Part model, mm, in its own coordinate system. Face numbers are marked on the shaded views. A direction names the side the tool comes from. Coordinates: 2 decimals unless noted, no trailing zeros. Write each loop counter-clockwise with the first axis right and the second up, starting at its lowest first coordinate (ties: lowest second). Pieces come first, ordered by that corner, then holes. Notation, with made-up numbers: (50.25, 56) - (89.25, 56) arc R19 ccw to (89.25, 78) - close; hole circle Ø11 at (53, 51.5). An arc over 180 degrees is marked (long way). Use a Markdown table: item, result.
```python
from build123d import *

# Parameters (mm, degrees)
F0_R     = 3.375
F0_R_2   = 20
F1_DEPTH = 15
F2_R     = 31.5
F3_DEPTH = 2
F4_SIZE  = 0.5
F5_SIZE  = 0.5
F6_R     = 23.75
F7_DEPTH = 2.25
F8_SIZE  = 1.5


with BuildPart() as f1:
    # F0 (on Top) → F1 (new body)
    with BuildSketch(Plane.XY):
        with BuildLine():
            ThreePointArc((-102.5, -0.229013), (-90.703842, -28.365124), (-62.500656, -40))
            Line((-62.500656, -40), (62.500656, -40))
            ThreePointArc((62.500656, -40), (90.703842, -28.365124), (102.5, -0.229013))
            Line((102.5, -0.229013), (102.5, 0.229013))
            ThreePointArc((102.5, 0.229013), (90.703842, 28.365124), (62.500656, 40))
            Line((62.500656, 40), (-62.500656, 40))
            ThreePointArc((-62.500656, 40), (-90.703842, 28.365124), (-102.5, 0.229013))
            Line((-102.5, 0.229013), (-102.5, -0.229013))
        make_face()
        with Locations((0, -25.125)):
            Circle(F0_R, mode=Mode.SUBTRACT)
        with Locations((-62.500656, 0)):
            Circle(F0_R_2, mode=Mode.SUBTRACT)
        with Locations((62.500656, 0)):
            Circle(F0_R_2, mode=Mode.SUBTRACT)
        with Locations((0, 25.125)):
            Circle(F0_R, mode=Mode.SUBTRACT)
        with BuildLine():
            ThreePointArc((-102.5, 0.229013), (-102.500656, 0), (-102.5, -0.229013))
            Line((-102.5, -0.229013), (-102.5, 0.229013))
        make_face()
        with BuildLine():
            Line((102.5, 0.229013), (102.5, -0.229013))
            ThreePointArc((102.5, -0.229013), (102.500656, 0), (102.5, 0.229013))
        make_face()
    extrude(amount=F1_DEPTH)

    # F2 (on face) → F3 (cut)
    with BuildSketch(Plane(origin=(0, 0, 0), x_dir=(1, 0, 0), z_dir=(0, 0, -1))):
        with Locations((-62.500656, 0)):
            Circle(F2_R)
        with Locations((62.500656, 0)):
            Circle(F2_R)
    extrude(amount=-F3_DEPTH, mode=Mode.SUBTRACT)

    # F4
    f4_edges = [f1.edges().sort_by_distance(p)[0] for p in [
        (62.500656, 40, 7.5),
        (-62.500656, 40, 7.5),
        (0, 40, 0),
        (0, 40, 15),
    ]]
    chamfer(f4_edges, length=F4_SIZE)

    # F5
    f5_edges = [f1.edges().sort_by_distance(p)[0] for p in [
        (-3.375, -25.125, 15),
        (-3.375, 25.125, 15),
        (-3.375, -25.125, 0),
        (-3.375, 25.125, 0),
    ]]
    chamfer(f5_edges, length=F5_SIZE)

    # F6 (on face) → F7 (cut)
    with BuildSketch(Plane.XY.offset(15)):
        with Locations((-62.500656, 0)):
            Circle(F6_R)
        with Locations((62.500656, 0)):
            Circle(F6_R)
    extrude(amount=-F7_DEPTH, mode=Mode.SUBTRACT)

    # F8
    f8_edges = [f1.edges().sort_by_distance(p)[0] for p in [
        (-82.500656, 0, 12.75),
        (42.500656, 0, 12.75),
    ]]
    chamfer(f8_edges, length=F8_SIZE)


solid = f1.part
```
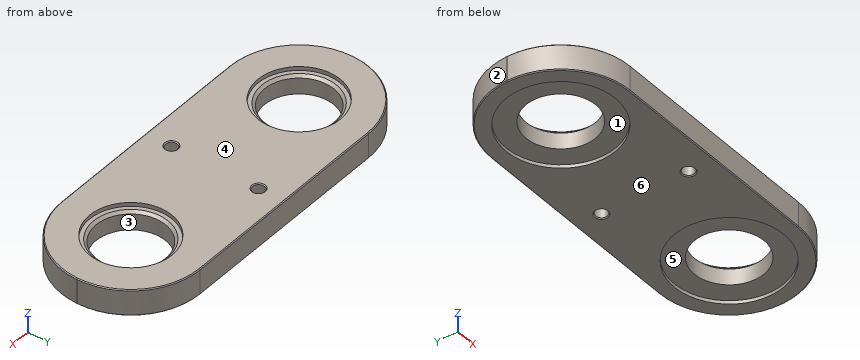
Item 1: Drop flat-ended pins along their axis: P1, Ø24, axis at x = 62.5, y = 0, coming from the +Z side; P2, Ø19, axis at x = 73.5, y = -13, coming from the -Z side; P3, Ø1.5, axis at x = -69, z = 4, coming from the +Y side; P4, Ø3, axis at y = -19.5, z = 2, coming from the -X side. Give the stop position or say it passes through.
From the geometry:
| item | result |
|---|---|
| P1 | through |
| P2 | z = 2 |
| P3 | y = 39.58 |
| P4 | x = -98.22 |
Item 2: Band-saw the part on B-B, the plane z = 9.25. Give the cut face in (x, y) (3 decimals).
From the geometry:
| item | result |
|---|---|
| outline | (-102.5, -0.229) arc R40 ccw to (-62.501, -40) - (62.501, -40) arc R40 ccw to (102.5, -0.229) arc R39.975 ccw to (102.5, 0.229) arc R40 ccw to (62.501, 40) - (-62.501, 40) arc R40 ccw to (-102.5, 0.229) arc R39.975 ccw to start; hole circle Ø40 at (-62.501, 0); hole circle Ø6.75 at (0, -25.125); hole circle Ø6.75 at (0, 25.125); hole circle Ø40 at (62.501, 0) |
Item 3: Band-saw the part on C-C, the plane y = -18. Count the separate pieces of the cut face and the enclosed holes in it, then the cut area to 3 significant figures.
From the geometry:
| item | result |
|---|---|
| separate pieces | 3 |
| enclosed holes | 0 |
| area | 2,220 mm^2 |
Item 4: Band-saw the part on A-A, the plane x = 0. Give the cut face in (y, z).
From the geometry:
| item | result |
|---|---|
| outline | (-40, 0.5) - (-39.5, 0) - (-29, 0) - (-28.5, 0.5) - (-28.5, 14.5) - (-29, 15) - (-39.5, 15) - (-40, 14.5) - close; (-21.75, 0.5) - (-21.25, 0) - (21.25, 0) - (21.75, 0.5) - (21.75, 14.5) - (21.25, 15) - (-21.25, 15) - (-21.75, 14.5) - close; (28.5, 0.5) - (29, 0) - (39.5, 0) - (40, 0.5) - (40, 14.5) - (39.5, 15) - (29, 15) - (28.5, 14.5) - close |
Item 5: Drill centre lines: probe 1 along X at (y, z) = (0, 0.7); probe 2 along X at (y, z) = (0, 5.25); probe 3 along Y at (x, z) = (-61.5, 10.25). Where is each one in solid material? Low to high.
From the geometry:
| item | result |
|---|---|
| probe 1 | -102.5 to -94, -31 to 31, 94 to 102.5 |
| probe 2 | -102.5 to -82.5, -42.5 to 42.5, 82.5 to 102.5 |
| probe 3 | -40 to -19.97, 19.97 to 40 |
Item 6: Which spindle directions (+Z, -Z, +X, -X, +Y, -Y) get a long thin tool onto all of the face, cutting with end or side? Do the marked faces 5 and 6. Say none if no direction does.
From the geometry:
| item | result |
|---|---|
| face 5 | -Z |
| face 6 | -Z, +X, -X, +Y, -Y |
Item 7: Two-plate mould, pull along Y, no slides. Class the marked faces 1, 2, 3 and 4: pulls with the +Y half, pulls with the -Y half, needs draft (parallel to the pull), parting line crosses it, or undercut.
From the geometry:
| item | result |
|---|---|
| face 1 | undercut |
| face 2 | pulls with the +Y half |
| face 3 | undercut |
| face 4 | needs draft |
